CAD build for the part. Positions are in the model's coordinates, mm. Give positions to 0.01 mm unless a question says otherwise; leave off trailing zeros. Write each loop counter-clockwise with the first axis right and the second up, starting at its lowest first coordinate (ties: lowest second). Pieces come first, ordered by that corner, then holes. Notation, with made-up numbers: (5, -2) - (33, -2) arc R22 ccw to (33, 31) - close; hole circle Ø5 at (31, -20). An arc over 180 degrees is marked (long way). Write item = value, one per line. Start each with the question number.
```python
from build123d import *

# Parameters (mm, degrees)
SKETCH_1_W             = 370
SKETCH_1_H             = 100
EXTRUDE_1_DEPTH        = 38
M12X1_25_1_D           = 10.5
PATTERN_LINEAR_1_COUNT = 2
PATTERN_LINEAR_1_PITCH = 90
PATTERN_LINEAR_3_COUNT = 2
PATTERN_LINEAR_3_PITCH = 150
PATTERN_LINEAR_4_COUNT = 2
PATTERN_LINEAR_4_PITCH = 210
PATTERN_LINEAR_5_COUNT = 2
PATTERN_LINEAR_5_PITCH = 300


with BuildPart() as part:
    # 草图1 → 凸台-拉伸1 (new body)
    with BuildSketch(Plane(origin=(0, 0, 0), x_dir=(1, 0, 0), z_dir=(0, 1, 0))):
        Rectangle(SKETCH_1_W, SKETCH_1_H)
    extrude(amount=EXTRUDE_1_DEPTH)

    # M12x1.25 螺纹孔1 (through all)
    with Locations(Plane(origin=(0, 38, 0), x_dir=(1, 0, 0), z_dir=(0, 1, 0))):
        with Locations((-150, 0)):
            m12x1_25_1 = Hole(M12X1_25_1_D / 2)

    # 阵列(线性)1: M12x1.25 螺纹孔1 ×2
    with Locations(*[(i * PATTERN_LINEAR_1_PITCH, 0, 0) for i in range(1, PATTERN_LINEAR_1_COUNT)]):
        add(m12x1_25_1, mode=Mode.SUBTRACT)

    # 阵列(线性)3: M12x1.25 螺纹孔1 ×2
    with Locations(*[(i * PATTERN_LINEAR_3_PITCH, 0, 0) for i in range(1, PATTERN_LINEAR_3_COUNT)]):
        add(m12x1_25_1, mode=Mode.SUBTRACT)

    # 阵列(线性)4: M12x1.25 螺纹孔1 ×2
    with Locations(*[(i * PATTERN_LINEAR_4_PITCH, 0, 0) for i in range(1, PATTERN_LINEAR_4_COUNT)]):
        add(m12x1_25_1, mode=Mode.SUBTRACT)

    # 阵列(线性)5: M12x1.25 螺纹孔1 ×2
    with Locations(*[(i * PATTERN_LINEAR_5_PITCH, 0, 0) for i in range(1, PATTERN_LINEAR_5_COUNT)]):
        add(m12x1_25_1, mode=Mode.SUBTRACT)


solid = part.part
```
1. Mould opens along Z. For faces 1 (the flat face through (-3, 19, -50)), 2 (the cylindrical face through (-54.755, 18.734, -0.231)), 3 (the cylindrical face through (145, 18.7, -1.6)), 4 (the flat face through (185, 19, 1)) say: +Z half, -Z half, draft (parallel to the pull), parting line (faces both ways), or undercut.
2. Cut at A-A (x = 60). Give the cut face in (y, z), then the cut area to 3 significant figures.
3. Cut at B-B (z = 0). Give the cut face in (x, y), then the cut area to 3 significant figures.
4. Wall check: line 1 along Z through (x, y) = (0, 13); line 2 along X through (y, z) = (15.5, -4); line 3 along Z through (x, y) = (154, 26). Give the ranges that are in metal, low to high.
5. Pin check, flat tip, straight feed: pin 1 Ø10 at (x, z) = (3, 19) entering from -Y. Stop position of the tip, or through.
Output:
q1.face_1 = -Z half
q1.face_2 = undercut
q1.face_3 = undercut
q1.face_4 = draft
q2.outline = (0, -50) - (38, -50) - (38, -5.25) - (0, -5.25) - close; (0, 5.25) - (38, 5.25) - (38, 50) - (0, 50) - close
q2.area = 3,400 mm2
q3.outline = (-185, 0) - (-155.25, 0) - (-155.25, 38) - (-185, 38) - close; (-144.75, 0) - (-65.25, 0) - (-65.25, 38) - (-144.75, 38) - close; (-54.75, 0) - (-5.25, 0) - (-5.25, 38) - (-54.75, 38) - close; (5.25, 0) - (54.75, 0) - (54.75, 38) - (5.25, 38) - close; (65.25, 0) - (144.75, 0) - (144.75, 38) - (65.25, 38) - close; (155.25, 0) - (185, 0) - (185, 38) - (155.25, 38) - close
q3.area = 12,100 mm2
q4.line_1 = -50 to -5.25, 5.25 to 50
q4.line_2 = -185 to -153.4, -146.6 to -63.4, -56.6 to -3.4, 3.4 to 56.6, 63.4 to 146.6, 153.4 to 185
q4.line_3 = -50 to -3.4, 3.4 to 50
q5.pin_1 = 0
